Here's how the part is built. I have some questions about the finished solid (model axes, mm). Round coordinates to 2 decimals unless told otherwise and drop trailing zeros. Order: outer loops, then holes, each group sorted by start corner. A loop starts at its lowest first (then second) coordinate and runs counter-clockwise, first axis right, second up.
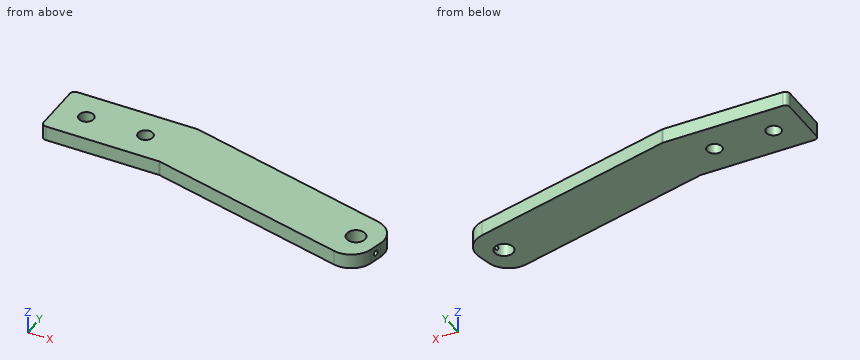
```python
from build123d import *

# Parameters (mm, degrees)
SKETCH1_R               = 3.175
SKETCH1_R_2             = 4
BOSS_EXTRUDE1_DEPTH     = 6.35
CUT_EXTRUDE2_REACH      = 155.866
CUT_EXTRUDE2_END_RADIUS = 4
SKETCH3_R               = 1.1303
FILLET3_R               = 2
FILLET4_R               = 10


with BuildPart() as part:
    # Sketch1 → Boss-Extrude1 (new body)
    with BuildSketch(Plane.XY):
        Polygon((-38.1, -12.7), (-38.1, 12.7), (15.701735639, 12.7), (114.28491418, -10.930870684), (108.364133554, -35.631161305), (12.7, -12.7), align=None)
        with Locations((-25.4, 0)):
            Circle(SKETCH1_R, mode=Mode.SUBTRACT)
        Circle(SKETCH1_R, mode=Mode.SUBTRACT)
        with Locations((101.6, -20.95)):
            Circle(SKETCH1_R_2, mode=Mode.SUBTRACT)
    extrude(amount=BOSS_EXTRUDE1_DEPTH)

    # Cut-Extrude2: up to this cylinder (the profile starts outside it)
    cut_extrude2_end = Plane(origin=(101.6, -20.95, 3.175), z_dir=(0, 0, -1)) * Cylinder(CUT_EXTRUDE2_END_RADIUS, 320.732, mode=Mode.PRIVATE)
    # Sketch3 → Cut-Extrude2 (cut, up to the surface)
    with BuildSketch(Plane(origin=(110.552900462, -26.500071647, 0), x_dir=(0, 0, -1), z_dir=(0.9724523866696595, -0.23310159943784806, 0)), mode=Mode.PRIVATE) as cut_extrude2_sk1:
        with Locations(Location((-3.175, 3.310245002, 0), (0, 0, 90))):
            Circle(SKETCH3_R)
    cut_extrude2_tool1 = extrude(cut_extrude2_sk1.sketch, amount=-CUT_EXTRUDE2_REACH, mode=Mode.PRIVATE) - cut_extrude2_end
    add(cut_extrude2_tool1.solids().sort_by_distance((111.324524, -23.281016, 3.175))[0], mode=Mode.SUBTRACT)

    # Fillet3
    fillet3_edges = [part.edges().sort_by_distance(p)[0] for p in [
        (12.7, -12.7, 3.175),
        (-38.1, -12.7, 3.175),
        (-38.1, 12.7, 3.175),
        (15.701735639, 12.7, 3.175),
    ]]
    fillet(fillet3_edges, radius=FILLET3_R)

    # Fillet4
    fillet4_edges = [part.edges().sort_by_distance(p)[0] for p in [
        (108.364133554, -35.631161305, 3.175),
        (114.28491418, -10.930870684, 3.175),
    ]]
    fillet(fillet4_edges, radius=FILLET4_R)


solid = part.part
```
1) I'm going to push flat-ended pins straight in: pin 1 (1.9 mm diameter, centred on x = 0, z = 3, fed in from -Y); pin 2 (1.5 mm diameter, centred on y = -28.5, z = 4.5, fed in from +X); pin 3 (10 mm diameter, centred on x = -25.4, y = 0, fed in from -Z); pin 4 (2 mm diameter, centred on x = 94, z = 2.5, fed in from +Y). Where does each tip first touch, or does it pass through?
2) If we section it at B-B (y = -18.5): Write out the boundary of the cut face in (x, z), plus the area to 3 significant figures.
3) I need wall thicknesses on line 1 (Y direction, x = -25.4, z = 3) (3 decimals); line 2 (Y direction, x = 12, z = 5.25); line 3 (Y direction, x = 101.6, z = 3.5). Which ranges of each line are inside material? Lowest first, please.
4) If we section it at C-C (y = 0): Write out the boundary of the cut face in (x, z) (3 decimals).
5) If we section it at D-D (x = 31): Write out the boundary of the cut face in (y, z), plus the area to 3 significant figures.
6) If we section it at A-A (x = -25.4): Write out the boundary of the cut face in (y, z) (3 decimals), plus the area to 3 significant figures.
Solutions:
1. pin 1: stops at y = -12.7
1. pin 2: stops at x = 110.06
1. pin 3: stops at z = 0
1. pin 4: stops at y = -5.83
2. outline: (36.9, 0) - (98.44, 0) - (98.44, 6.35) - (36.9, 6.35) - close; (104.76, 0) - (112.23, 0) - (112.23, 6.35) - (104.76, 6.35) - close
2. area: 438 mm2
3. line 1: y = -12.7 to -3.175, 3.175 to 12.7
3. line 2: y = -12.7 to 12.7
3. line 3: y = -33.56 to -24.95, -16.95 to -7.89
4. outline: (-38.1, 0) - (-28.575, 0) - (-28.575, 6.35) - (-38.1, 6.35) - close; (-22.225, 0) - (-3.175, 0) - (-3.175, 6.35) - (-22.225, 6.35) - close; (3.175, 0) - (68.684, 0) - (68.684, 6.35) - (3.175, 6.35) - close
5. outline: (-17.09, 0) - (9.03, 0) - (9.03, 6.35) - (-17.09, 6.35) - close
5. area: 166 mm2
6. outline: (-12.7, 0) - (-3.175, 0) - (-3.175, 6.35) - (-12.7, 6.35) - close; (3.175, 0) - (12.7, 0) - (12.7, 6.35) - (3.175, 6.35) - close
6. area: 121 mm2
